The drawing under review shows one solid part. Ordinate dimensions are in mm from its lowest x, y, z. Give positions to 0.01 mm unless a question says otherwise; leave off trailing zeros. Order: outer loops, then holes, each group sorted by start corner. A loop starts at its lowest first (then second) coordinate and runs counter-clockwise, first axis right, second up. Notation, with made-up numbers: (22.5, -31.75) - (46.5, -31.75) arc R17 cw to (46.5, -14.75) - close; hole circle Ø1 at (29.25, 20.5). An arc over 180 degrees is marked (long way). Use CSV: the item, a comma, the result in double quotes.
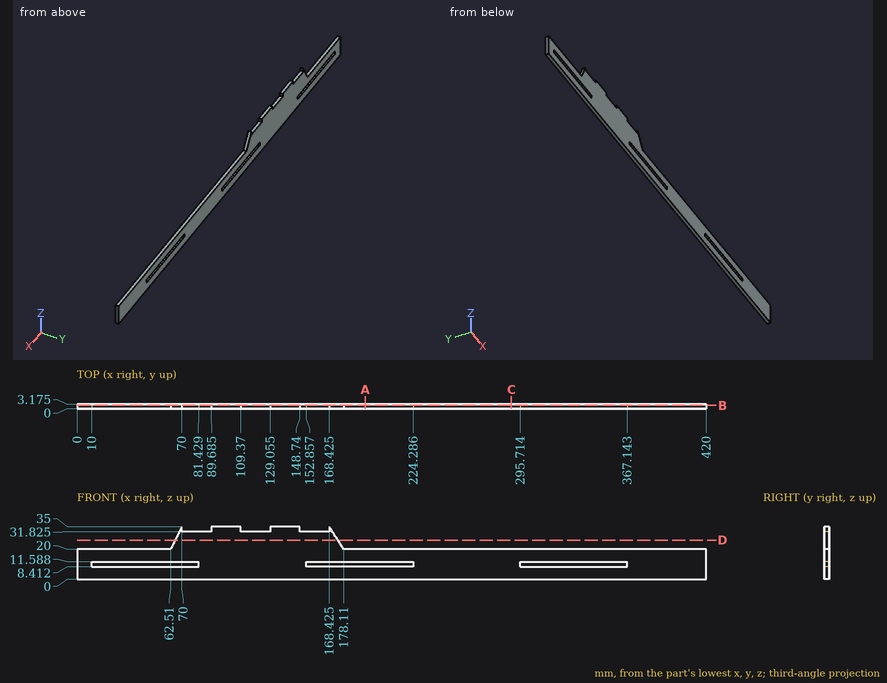
Item 1: Clearance check with flat-ended pins moving along their axes: pin 1 (1.6 mm diameter, centred on y = 1.5, z = 34, fed in from +X); pin 2 (1.6 mm diameter, centred on x = 31.5, y = 2, fed in from +Z); pin 3 (1 mm diameter, centred on y = 2, z = 33.5, fed in from +X) (1 decimal). State where each tip first meets the part, or that it passes through.
Results list:
pin 1,"stops at x = 169.59"
pin 2,"stops at z = 20"
pin 3,"stops at x = 169.7"
Item 2: Take a section at C-C, the plane x = 290. Give the boundary of the cut face in (y, z) (1 decimal).
Results list:
outline,"(0, 0) - (3.2, 0) - (3.2, 20) - (0, 20) - close"
Item 3: Take a section at A-A, the plane x = 192.5. Give the boundary of the cut face in (y, z) (1 decimal).
Results list:
outline,"(0, 0) - (3.2, 0) - (3.2, 8.4) - (0, 8.4) - close; (0, 11.6) - (3.2, 11.6) - (3.2, 20) - (0, 20) - close"
Item 4: Take a section at D-D, the plane z = 26. Give the boundary of the cut face in (x, y) (1 decimal), and give its area (3 significant figures).
Results list:
outline,"(65.5, 0) - (174.2, 0) - (174.2, 3.2) - (65.5, 3.2) - close"
area,"345 mm2"
Item 5: Wall thickness on L1, parallel to X at y = 0.95, z = 9 (1 decimal); L2, parallel to Z at x = 206, y = 1; L3, parallel to X at y = 0.35, z = 32 (1 decimal): over which ranges is each line inside the solid? List them lowest first.
Results list:
L1,"x = 0 to 10, 81.4 to 152.9, 224.3 to 295.7, 367.1 to 420"
L2,"z = 0 to 8.41, 11.59 to 20"
L3,"x = 68.5 to 70, 89.7 to 109.4, 129.1 to 148.7, 168.4 to 170.4"
Item 6: Take a section at B-B, the plane y = 2.2. State how many separate pieces and enclosed holes the cut face has, and give its area (3 significant figures).
Results list:
separate pieces,"1"
enclosed holes,"3"
area,"9,140 mm2"
